Geometry check sheet. Reference: the model listing, model coordinates, mm. Face numbers are marked on the shaded views. A direction names the side the tool comes from. Coordinates: 2 decimals unless noted, no trailing zeros. Order: outer loops, then holes, each group sorted by start corner. A loop starts at its lowest first (then second) coordinate and runs counter-clockwise, first axis right, second up. Notation, with made-up numbers: (61, 66) - (77, 66) arc R8 ccw to (77, 73) - close; hole circle Ø8 at (5.25, -17.5). An arc over 180 degrees is marked (long way). Return JSON: item names as keys, results as strings. Group by question number.
Item 1: Section check D-D on y = 0.5. Enter the section's corners in (x, z).
Item 2: Section check C-C on y = 5.25. Enter the section's corners in (x, z).
Item 3: Gauge pin test, flat ends, axial feed: pin 1 (1.6 mm diameter, centred on y = 0.5, z = 10, fed in from +X); pin 2 (1 mm diameter, centred on y = 2, z = -9.5, fed in from -X); pin 3 (2 mm diameter, centred on x = 0, z = -10.5, fed in from -Y); pin 4 (2 mm diameter, centred on x = -1, z = 10, fed in from +Y). Record the tip position at first contact, or that the pin passes through.
Item 4: Section check B-B on x = 0. Enter the section's corners in (y, z).
Item 5: Section check A-A on z = -10.5. Enter the section's corners in (x, y).
Item 6: Scan lines: probe 1 along Z at (x, y) = (2.25, 1.25); probe 2 along Z at (x, y) = (0, 3.25); probe 3 along X at (y, z) = (6.95, 0). Record each from-to range of solid material in increasing order.
Item 7: Draft check along X on the marked faces 4, 5 and 6. Enter one of: pulls with the +X half, pulls with the -X half, needs draft (parallel to the pull), parting line crosses it, or undercut.
Item 8: Tool access check on the marked faces 1, 2 and 3. Record the directions out of +Z, -Z, +X, -X, +Y, -Y that give a thin tool (end or side, any length) a straight path to the whole face; none if there is none.
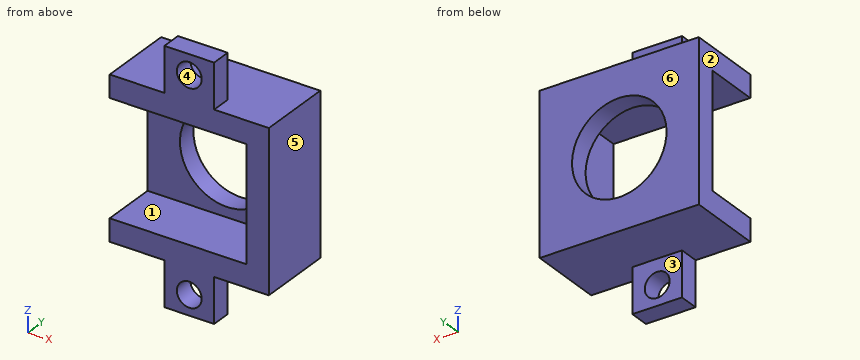
from build123d import *

# Parameters (mm, degrees)
SKETCH1_W           = 16
SKETCH1_H           = 16
BOSS_EXTRUDE1_DEPTH = 7.6
SKETCH2_W           = 11.5
SKETCH2_H           = 11.5
CUT_EXTRUDE1_DEPTH  = 5.6
SKETCH3_W           = 2.25
SKETCH3_H           = 11.5
CUT_EXTRUDE2_DEPTH  = 5.6
SKETCH4_R           = 4.75
CUT_EXTRUDE3_DEPTH  = 7.6
SKETCH5_W           = 5
SKETCH5_H           = 4.5
BOSS_EXTRUDE2_DEPTH = 2
CUT_EXTRUDE4_REACH  = 17.862
SKETCH6_R           = 1.25


with BuildPart() as part:
    # Sketch1 → Boss-Extrude1 (new body)
    with BuildSketch(Plane(origin=(0, 0, 0), x_dir=(1, 0, 0), z_dir=(0, 1, 0))):
        Rectangle(SKETCH1_W, SKETCH1_H)
    extrude(amount=BOSS_EXTRUDE1_DEPTH)

    # Sketch2 → Cut-Extrude1 (cut)
    with BuildSketch(Plane(origin=(0, 0, 0), x_dir=(1, 0, 0), z_dir=(0, 1, 0))):
        Rectangle(SKETCH2_W, SKETCH2_H)
    extrude(amount=CUT_EXTRUDE1_DEPTH, mode=Mode.SUBTRACT)

    # Sketch3 → Cut-Extrude2 (cut)
    with BuildSketch(Plane.XZ):
        with Locations((-6.875, 0)):
            Rectangle(SKETCH3_W, SKETCH3_H)
    extrude(amount=-CUT_EXTRUDE2_DEPTH, mode=Mode.SUBTRACT)

    # Sketch4 → Cut-Extrude3 (cut)
    with BuildSketch(Plane(origin=(0, 7.6, 0), x_dir=(1, 0, 0), z_dir=(0, 1, 0))):
        with Locations(Location((0, 0, 0), (0, 0, 270))):
            Circle(SKETCH4_R)
    extrude(amount=-CUT_EXTRUDE3_DEPTH, mode=Mode.SUBTRACT)

    # Sketch5 → Boss-Extrude2 (add)
    with BuildSketch(Plane(origin=(0, 0, 0), x_dir=(1, 0, 0), z_dir=(0, 1, 0))):
        with Locations((0, 10.25)):
            Rectangle(SKETCH5_W, SKETCH5_H)
    boss_extrude2 = extrude(amount=BOSS_EXTRUDE2_DEPTH)

    # Sketch6 → Cut-Extrude4 (cut, up to next)
    with BuildSketch(Plane(origin=(0, 2, 0), x_dir=(1, 0, 0), z_dir=(0, 1, 0)), mode=Mode.PRIVATE) as cut_extrude4_sk1:
        with Locations(Location((0, 10.5, 0), (0, 0, 270))):
            Circle(SKETCH6_R)
    cut_extrude4_tool1 = extrude(cut_extrude4_sk1.sketch, amount=-CUT_EXTRUDE4_REACH, mode=Mode.PRIVATE) & part.part
    cut_extrude4 = cut_extrude4_tool1.solids().sort_by_distance((0, 2, -10.5))[0]
    add(cut_extrude4, mode=Mode.SUBTRACT)

    # Mirror1: Boss-Extrude2, Cut-Extrude4 across plane
    add(boss_extrude2.mirror(Plane.XY))
    add(cut_extrude4.mirror(Plane.XY), mode=Mode.SUBTRACT)


solid = part.part
Computed:
{
 "1": {"outline": "(-8, -8) - (-2.5, -8) - (-2.5, -12.5) - (2.5, -12.5) - (2.5, -8) - (8, -8) - (8, 8) - (2.5, 8) - (2.5, 12.5) - (-2.5, 12.5) - (-2.5, 8) - (-8, 8) - (-8, 5.75) - (5.75, 5.75) - (5.75, -5.75) - (-8, -5.75) - close; hole circle Ø2.5 at (0, -10.5); hole circle Ø2.5 at (0, 10.5)"},
 "2": {"outline": "(-8, -8) - (8, -8) - (8, 8) - (-8, 8) - (-8, 5.75) - (5.75, 5.75) - (5.75, -5.75) - (-8, -5.75) - close"},
 "3": {"pin 1": "stops at x = 2.5", "pin 2": "stops at x = -2.5", "pin 3": "passes through", "pin 4": "stops at y = 2"},
 "4": {"outline": "(0, -12.5) - (2, -12.5) - (2, -11.75) - (0, -11.75) - close; (0, -9.25) - (2, -9.25) - (2, -8) - (7.6, -8) - (7.6, -4.75) - (5.6, -4.75) - (5.6, -5.75) - (0, -5.75) - close; (0, 5.75) - (5.6, 5.75) - (5.6, 4.75) - (7.6, 4.75) - (7.6, 8) - (2, 8) - (2, 9.25) - (0, 9.25) - close; (0, 11.75) - (2, 11.75) - (2, 12.5) - (0, 12.5) - close"},
 "5": {"outline": "(-2.5, 0) - (-1.25, 0) - (-1.25, 2) - (-2.5, 2) - close; (1.25, 0) - (2.5, 0) - (2.5, 2) - (1.25, 2) - close"},
 "6": {"probe 1": "z = -12.5 to -5.75, 5.75 to 12.5", "probe 2": "z = -8 to -5.75, 5.75 to 8", "probe 3": "x = -8 to -4.75, 4.75 to 8"},
 "7": {"face 4": "undercut", "face 5": "pulls with the +X half", "face 6": "needs draft"},
 "8": {"face 1": "-X, -Y", "face 2": "+Z, -Z, -X, +Y, -Y", "face 3": "-Z, +X, -X, +Y"}
}
